from build123d import *

# Parameters (mm, degrees)
BOSS_EXTRUDE1_START     = -445.39
BOSS_EXTRUDE1_OUTLINE_W = 89.79
BOSS_EXTRUDE1_OUTLINE_H = 11.81
BOSS_EXTRUDE1_DEPTH     = 585.980036335
JOINT_X_W               = 25.4
JOINT_X_H               = 11.81
BOSS_EXTRUDE2_DEPTH     = 11.81
LPATTERN1_COUNT         = 3
LPATTERN1_PITCH         = 280.290018167
JOINT_Y_W               = 11.81
JOINT_Y_H               = 25.4
BOSS_EXTRUDE3_DEPTH     = 11.81
LPATTERN2_COUNT         = 3
LPATTERN2_PITCH         = 38.1
MIRROR3_COPY_1_SKETCH_W = 11.81
MIRROR3_COPY_1_SKETCH_H = 25.4
MIRROR3_COPY_1_DEPTH    = 11.81
MIRROR3_COPY_2_SKETCH_W = 11.81
MIRROR3_COPY_2_SKETCH_H = 25.4
MIRROR3_COPY_2_DEPTH    = 11.81


# Read off the part's stored shape, not the designer's step: Boss-Extrude1
with BuildPart() as part:
    # Boss-Extrude1 outline → Boss-Extrude1 (new body)
    with BuildSketch(Plane.YZ.offset(BOSS_EXTRUDE1_START)):
        with Locations((52.039215162, 5.905)):
            Rectangle(BOSS_EXTRUDE1_OUTLINE_W, BOSS_EXTRUDE1_OUTLINE_H)
    extrude(amount=BOSS_EXTRUDE1_DEPTH)

    # Joint_X → Boss-Extrude2 (add)
    with BuildSketch(Plane.XY.offset(11.81)):
        with Locations((-432.69, 1.239215162)):
            Rectangle(JOINT_X_W, JOINT_X_H)
    boss_extrude2 = extrude(amount=-BOSS_EXTRUDE2_DEPTH)

    # LPattern1: Boss-Extrude2 ×3
    with Locations(*[(i * LPATTERN1_PITCH, 0, 0) for i in range(1, LPATTERN1_COUNT)]):
        add(boss_extrude2)

    # Joint_Y → Boss-Extrude3 (add)
    with BuildSketch(Plane.XY.offset(11.81)):
        with Locations((-451.295, 8.034215162)):
            Rectangle(JOINT_Y_W, JOINT_Y_H)
    boss_extrude3 = extrude(amount=-BOSS_EXTRUDE3_DEPTH)

    # LPattern2: Boss-Extrude3 ×3
    with Locations(*[(0, i * LPATTERN2_PITCH, 0) for i in range(1, LPATTERN2_COUNT)]):
        add(boss_extrude3)

    # Mirror3: Boss-Extrude3 across plane
    add(boss_extrude3.mirror(Plane.ZY.offset(152.399981833)))

    # Mirror3 copy 1 sketch → Mirror3 copy 1 (add)
    with BuildSketch(Plane(origin=(-304.799963665, 38.1, 11.81), x_dir=(-1, 0, 0), z_dir=(0, 0, 1))):
        with Locations((-451.295, -8.034215162)):
            Rectangle(MIRROR3_COPY_1_SKETCH_W, MIRROR3_COPY_1_SKETCH_H)
    extrude(amount=-MIRROR3_COPY_1_DEPTH)

    # Mirror3 copy 2 sketch → Mirror3 copy 2 (add)
    with BuildSketch(Plane(origin=(-304.799963665, 76.2, 11.81), x_dir=(-1, 0, 0), z_dir=(0, 0, 1))):
        with Locations((-451.295, -8.034215162)):
            Rectangle(MIRROR3_COPY_2_SKETCH_W, MIRROR3_COPY_2_SKETCH_H)
    extrude(amount=-MIRROR3_COPY_2_DEPTH)


solid = part.part
The listing builds one solid part. Answer for the finished solid, in the listing's coordinates (mm). A direction names the side the tool comes from. Round coordinates to 2 decimals unless told otherwise and drop trailing zeros. Order: outer loops, then holes, each group sorted by start corner. A loop starts at its lowest first (then second) coordinate and runs counter-clockwise, first axis right, second up. Notation, with made-up numbers: (-11, 53.5) - (22, 53.5) arc R18 ccw to (22, 82.5) - close; hole circle Ø5 at (39.5, 87). An arc over 180 degrees is marked (long way). Write item = value, one per line. Start each with the question number.
1) Section B-B, the plane x = 37.5 is taken. Write down the section's boundary in (y, z), plus the area to 3 significant figures.
2) Section A-A, the plane z = 4.25 is taken. Write down the section's boundary in (x, y).
3) For faces 1 (the flat face through (140.59, 65, 6)), 2 (the flat face through (-451, 58.834, 6)), 3 (the flat face through (-457.2, 8, 6)), 4 (the flat face through (-419.99, 1, 6)), 5 (the flat face through (134, -4.666, 6)), determine the directions among +Z, -Z, +X, -X, +Y, -Y from which every point of the face is accessible in a straight line to the end or side of a thin tool.
4) For a pull along Y with two mould halves and no side action, classify faces 6 (the flat face through (115.19, 1, 6)), 7 (the flat face through (147, 33.434, 6)), 8 (the flat face through (-148, 96.934, 6)), 9 (the flat face through (-294, 7.144, 6)) as released by +Y, released by -Y, zero draft, split by the parting line, or undercut.
5) Given pin 1 (3.5 mm diameter, centred on x = 13.5, z = 5.5, fed in from -Y); pin 2 (5 mm diameter, centred on y = 67.5, z = 10, fed in from +X); pin 3 (6 mm diameter, centred on x = 41.5, y = 21.5, fed in from -Z), each flat-ended and moving along its own axis, determine where each tip first touches the part or whether it passes through.
6) Straight lines are drawn through the part: L1, parallel to X at y = 5.5, z = 3.75; L2, parallel to Y at x = -256, z = 1; L3, parallel to X at y = 23.5, z = 11. For each, find the intervals that lie inside material, in ascending order.
Results list:
q1.outline = (7.14, 0) - (96.93, 0) - (96.93, 11.81) - (7.14, 11.81) - close
q1.area = 1,060 mm^2
q2.outline = (-457.2, -4.67) - (-419.99, -4.67) - (-419.99, 7.14) - (-165.1, 7.14) - (-165.1, -4.67) - (-139.7, -4.67) - (-139.7, 7.14) - (115.19, 7.14) - (115.19, -4.67) - (152.4, -4.67) - (152.4, 20.73) - (140.59, 20.73) - (140.59, 33.43) - (152.4, 33.43) - (152.4, 58.83) - (140.59, 58.83) - (140.59, 71.53) - (152.4, 71.53) - (152.4, 96.93) - (-457.2, 96.93) - (-457.2, 71.53) - (-445.39, 71.53) - (-445.39, 58.83) - (-457.2, 58.83) - (-457.2, 33.43) - (-445.39, 33.43) - (-445.39, 20.73) - (-457.2, 20.73) - close
q3.face_1 = +Z, -Z, +X
q3.face_2 = +Z, -Z, -X
q3.face_3 = +Z, -Z, -X, +Y, -Y
q3.face_4 = +Z, -Z, -Y
q3.face_5 = +Z, -Z, +X, -X, -Y
q4.face_6 = zero draft
q4.face_7 = undercut
q4.face_8 = released by +Y
q4.face_9 = released by -Y
q5.pin_1 = 7.14
q5.pin_2 = 140.59
q5.pin_3 = 0
q6.L1 = -457.2 to -419.99, -165.1 to -139.7, 115.19 to 152.4
q6.L2 = 7.14 to 96.93
q6.L3 = -445.39 to 140.59
